Here's how the part is built. I have some questions about the finished solid (model axes, mm). A direction names the side the tool comes from. Round coordinates to 2 decimals unless told otherwise and drop trailing zeros. Order: outer loops, then holes, each group sorted by start corner. A loop starts at its lowest first (then second) coordinate and runs counter-clockwise, first axis right, second up. Notation, with made-up numbers: (40.5, 10.5) - (93.5, 10.5) arc R24 cw to (93.5, 25.5) - close; hole circle Ø11 at (73, -39.5). An arc over 180 degrees is marked (long way). One line per item, written item: value.
from build123d import *

# Parameters (mm, degrees)
F0_W     = 98
F0_H     = 95
F1_DEPTH = 3
F2_R     = 36.25
F2_R_2   = 33.25
F3_DEPTH = 4
F4_R     = 36.25
F4_R_2   = 34.5
F5_DEPTH = 60
F6_W     = 94.875
F6_H     = 94.875
F6_W_2   = 92
F6_H_2   = 92
F7_DEPTH = 10


with BuildPart() as f1:
    # F0 (on Front) → F1 (new body)
    with BuildSketch(Plane.XZ):
        Rectangle(F0_W, F0_H)
    extrude(amount=-F1_DEPTH)

    # F2 (on Front) → F3 (cut)
    with BuildSketch(Plane.XZ):
        with Locations((0, 8.75)):
            Circle(F2_R)
        with Locations((0, 8.75)):
            Circle(F2_R_2, mode=Mode.SUBTRACT)
        with Locations((0, 8.75)):
            Circle(F2_R_2)
    extrude(amount=-F3_DEPTH, mode=Mode.SUBTRACT)

    # F4 (on face) → F5 (join)
    with BuildSketch(Plane.XZ):
        with Locations((0, 8.75)):
            Circle(F4_R)
        with Locations((0, 8.75)):
            Circle(F4_R_2, mode=Mode.SUBTRACT)
    extrude(amount=-F5_DEPTH)

    # F6 (on Front) → F7 (join)
    with BuildSketch(Plane.XZ):
        Rectangle(F6_W, F6_H)
        Rectangle(F6_W_2, F6_H_2, mode=Mode.SUBTRACT)
    extrude(amount=F7_DEPTH)


solid = f1.part
Q1. Which directions (+Z, -Z, +X, -X, +Y, -Y) give clear straight access to the entire face, cutting with the end or side of a thin tool? Please do faces 4 (the flat face through (49, 1, -1)), 5 (the flat face through (-1, 3, -31)), 6 (the cylindrical face through (-7.48, 29.58, -24.93)), 7 (the flat face through (-46, -5, -1)), 8 (the flat face through (-47.438, -5, -1)).
Results list:
face 4: +Z, -Z, +X, +Y, -Y
face 5: +Y
face 6: +Y, -Y
face 7: -Y
face 8: +Z, -Z, -X, -Y
Q2. If we section it at B-B, the plane z = 8.75: Please give me the cut outline in (x, y).
Results list:
outline: (-49, 0) - (-47.44, 0) - (-47.44, -10) - (-46, -10) - (-46, 0) - (-34.5, 0) - (-34.5, 60) - (-36.25, 60) - (-36.25, 3) - (-49, 3) - close; (34.5, 0) - (46, 0) - (46, -10) - (47.44, -10) - (47.44, 0) - (49, 0) - (49, 3) - (36.25, 3) - (36.25, 60) - (34.5, 60) - close
Q3. If we section it at C-C, the plane x = 0: Please give me the cut outline in (y, z), then the cut area to 3 significant figures.
Results list:
outline: (-10, -47.44) - (0, -47.44) - (0, -47.5) - (3, -47.5) - (3, -27.5) - (60, -27.5) - (60, -25.75) - (0, -25.75) - (0, -46) - (-10, -46) - close; (-10, 46) - (0, 46) - (0, 43.25) - (60, 43.25) - (60, 45) - (3, 45) - (3, 47.5) - (0, 47.5) - (0, 47.44) - (-10, 47.44) - close
area: 306 mm²
Q4. If we section it at D-D, the plane x = -41: Please give me the cut outline in (y, z), then the cut area to 3 significant figures.
Results list:
outline: (-10, -47.44) - (0, -47.44) - (0, -47.5) - (3, -47.5) - (3, 47.5) - (0, 47.5) - (0, 47.44) - (-10, 47.44) - (-10, 46) - (0, 46) - (0, -46) - (-10, -46) - close
area: 314 mm²
Q5. We'd pull the mould along Z, two halves only. Please class faces 1 (the flat face through (-1, 1, 47.5)), 2 (the flat face through (32, 60, -5)), 3 (the flat face through (-1, -5, 46)): released by +Z, released by -Z, zero draft, split by the parting line, or undercut.
Results list:
face 1: released by +Z
face 2: zero draft
face 3: undercut
Q6. If I drill on line 1 along Z through (x, y) = (-14.5, -5); line 2 along Z through (x, y) = (0, 27), over which ranges is the centre line in solid material (lowest first)?
Results list:
line 1: -47.44 to -46, 46 to 47.44
line 2: -27.5 to -25.75, 43.25 to 45
Q7. Will these pins go through, and if not, where does the flat tip stop? pin 1 (3 mm diameter, centred on x = -16.5, y = -6.5, fed in from +Z); pin 2 (8 mm diameter, centred on y = -6.5, z = -14, fed in from +X); pin 3 (8 mm diameter, centred on y = -7, z = -19.5, fed in from -X); pin 4 (12 mm diameter, centred on x = 1.5, z = -14, fed in from -Y).
Results list:
pin 1: z = 47.44
pin 2: x = 47.44
pin 3: x = -47.44
pin 4: through
Q8. If we section it at A-A, the plane y = -5: Please give me the cut outline in (x, z), then the cut area to 3 significant figures.
Results list:
outline: (-47.44, -47.44) - (47.44, -47.44) - (47.44, 47.44) - (-47.44, 47.44) - close; hole (-46, -46) - (46, -46) - (46, 46) - (-46, 46) - close
area: 537 mm²
